Can you work these out from the model? Positions are in its coordinate system, mm. Face numbers are marked on the shaded views. Give positions to 0.01 mm unless a question says otherwise; leave off trailing zeros. Write each loop counter-clockwise with the first axis right and the second up, starting at its lowest first coordinate (ties: lowest second). Pieces come first, ordered by that corner, then holes. Notation, with made-up numbers: (57.5, -23) -> (71.5, -23) arc R10 cw to (71.5, -10) -> close; hole circle Ø2 at (79.25, 13.25). An arc over 180 degrees is marked (long way). Answer as CSV lines item,"result". Start each with the question number.
1. I need wall thicknesses on line 1 (X direction, y = 3, z = 5.5); line 2 (X direction, y = 5, z = 7); line 3 (Y direction, x = 5, z = 4.25). Which ranges of each line are inside material? Lowest first, please. Write a range as [from, to].
2. If we section it at B-B on z = 4.75: Write out the boundary of the cut face in (x, y), plus the area to 3 significant figures.
3. I'm going to push flat-ended pins straight in: P1, Ø3, axis at y = 9, z = 4.5, coming from the -X side; P2, Ø2, axis at y = -10.5, z = 1, coming from the +X side; P3, Ø1.5, axis at x = -4.5, y = 2, coming from the +Z side. Where does each tip first touch, or does it pass through?
4. If we mould it in two halves opening along X, with no side actions, what happens to the marked faces 1, 2, 3 and 4? For each: pulls with the +X half, pulls with the -X half, needs draft (parallel to the pull), parting line crosses it, or undercut.
5. If we section it at A-A on y = 0: Write out the boundary of the cut face in (x, z).
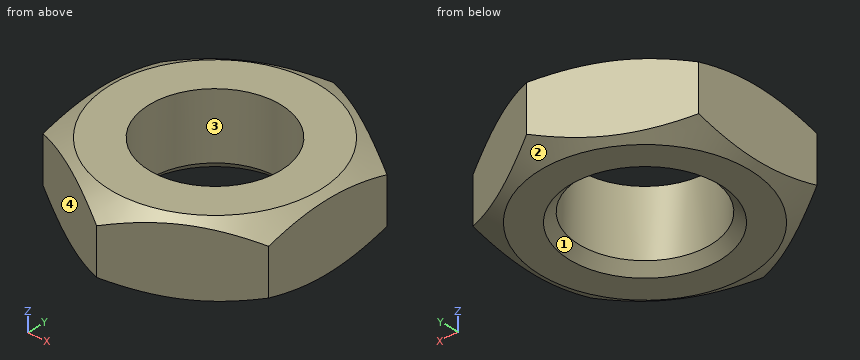
```python
from build123d import *

# Parameters (mm, degrees)
SKETCH_1_R      = 7
EXTRUDE_1_DEPTH = 8
CHAMFER_1_SIZE  = 1


with BuildPart() as part:
    # Эскиз1 → Бобышка-Вытянуть1 (new body)
    with BuildSketch(Plane.XY):
        Polygon((0, 13.856406461), (-12, 6.92820323), (-12, -6.92820323), (0, -13.856406461), (12, -6.92820323), (12, 6.92820323), align=None)
        Circle(SKETCH_1_R, mode=Mode.SUBTRACT)
    extrude(amount=EXTRUDE_1_DEPTH)

    # Эскиз2 → Вырез-Повернуть1 (revolve, cut)
    with BuildSketch(Plane(origin=(0, 0, 0), x_dir=(0, 0, -1), z_dir=(1, 0, 0)), mode=Mode.PRIVATE) as cut_revolve_1_sk:
        Polygon((0, 13.856406461), (-1.562544499, 13.856406461), (0, 11.15), align=None)
        Polygon((-8, 11.15), (-8, 13.856406461), (-6.437455501, 13.856406461), align=None)
    revolve(cut_revolve_1_sk.sketch.rotate(Axis((0, 0, 0), (0, 0, 1)), 90), axis=Axis((0, 0, 0), (0, 0, 1)), mode=Mode.SUBTRACT)

    # Фаска1
    chamfer_1_edges = [part.edges().sort_by_distance(p)[0] for p in [
        (-7, 0, 0),
    ]]
    chamfer(chamfer_1_edges, length=CHAMFER_1_SIZE)


solid = part.part
```
Computed values:
1,line 1,"x = [-12, -6.32], [6.32, 12]"
1,line 2,"x = [-11.87, -4.9], [4.9, 11.87]"
1,line 3,"y = [-10.97, -4.9], [4.9, 10.97]"
2,outline,"(-12, -6.93) -> (0, -13.86) -> (12, -6.93) -> (12, 6.93) -> (0, 13.86) -> (-12, 6.93) -> close; hole circle Ø14 at (0, 0)"
2,area,"345 mm2"
3,P1,"stops at x = -11.01"
3,P2,"stops at x = 7.55"
3,P3,"passes through"
4,face 1,"undercut"
4,face 2,"parting line crosses it"
4,face 3,"undercut"
4,face 4,"pulls with the -X half"
5,outline,"(-12, 0.49) -> (-11.15, 0) -> (-8, 0) -> (-7, 1) -> (-7, 8) -> (-11.15, 8) -> (-12, 7.51) -> close; (7, 1) -> (8, 0) -> (11.15, 0) -> (12, 0.49) -> (12, 7.51) -> (11.15, 8) -> (7, 8) -> close"
